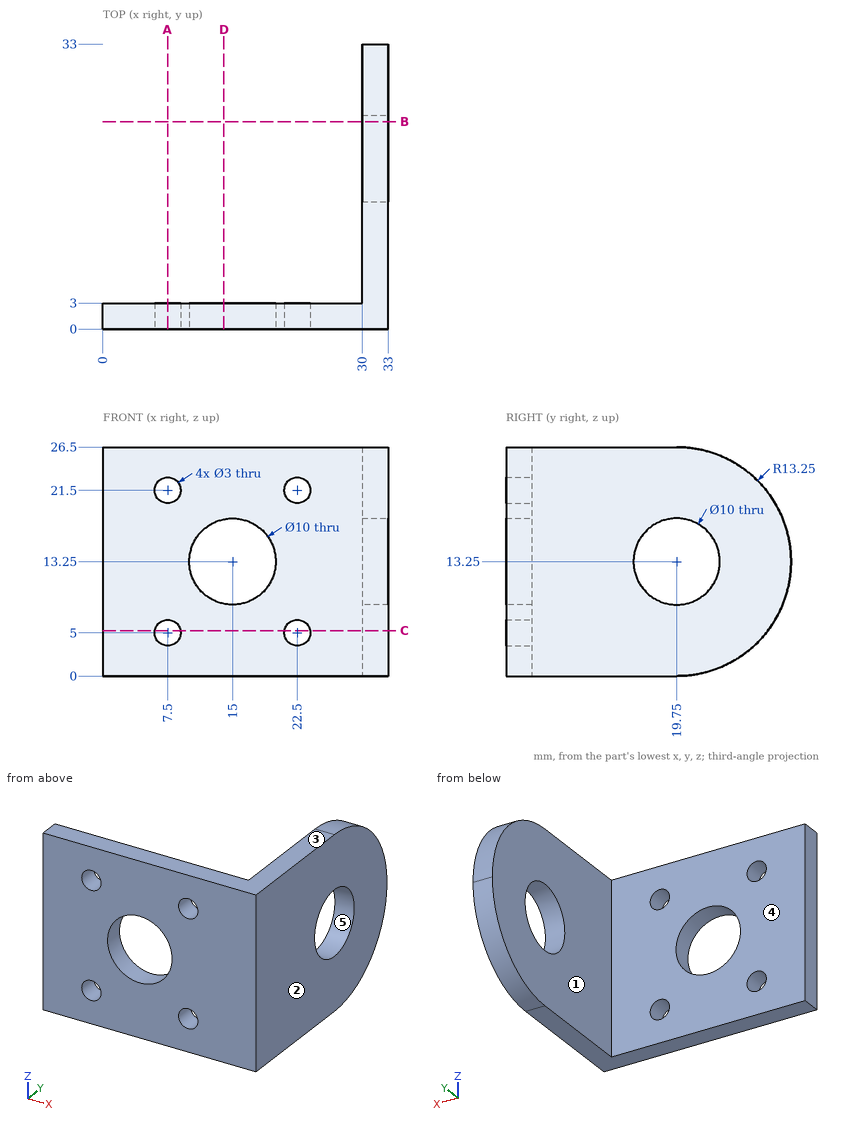
Part print with two shaded views. Sizes in mm from the minimum x, y, z corner. A direction names the side the tool comes from. Coordinates: 2 decimals unless noted, no trailing zeros. Write each loop counter-clockwise with the first axis right and the second up, starting at its lowest first coordinate (ties: lowest second). Pieces come first, ordered by that corner, then holes. Notation, with made-up numbers: (55.25, 68.25) - (70.25, 68.25) arc R16 cw to (70.25, 73.25) - close; hole circle Ø6 at (-20, 58). An arc over 180 degrees is marked (long way). Put each result on its own line as item: value.
1. Band-saw the part on D-D (x = 14). Write the cut outline in (y, z), then the cut area to 3 significant figures.
Final values:
outline: (0, 0) - (3, 0) - (3, 8.35) - (0, 8.35) - close; (0, 18.15) - (3, 18.15) - (3, 26.5) - (0, 26.5) - close
area: 50.1 mm²
2. Flat gauge pins, fed straight in: pin 1 Ø10 at (y, z) = (17, 11.5) entering from -X; pin 2 Ø8 at (y, z) = (19.75, 13.25) entering from -X; pin 3 Ø3 at (x, z) = (12, 8.5) entering from -Y; pin 4 Ø8 at (x, z) = (19.5, 10) entering from +Y. Where does each tip first touch, or does it go through?
Final values:
pin 1: stops at x = 30
pin 2: passes through
pin 3: stops at y = 0
pin 4: stops at y = 3
3. 3-axis set-ups, long thin cutter, end or side, ignore diameter. For the marked faces 1 and 2: which of +Z, -Z, +X, -X, +Y, -Y reach the whole face in a straight line?
Final values:
face 1: +Z, -Z, -X, +Y
face 2: +Z, -Z, +X, +Y, -Y
4. Two-plate mould, pull along Z, no slides. Class the marked faces 3, 4 and 5: +Z half, -Z half, draft (parallel to the pull), parting line (faces both ways), or undercut.
Final values:
face 3: +Z half
face 4: draft
face 5: undercut
5. Band-saw the part on C-C (z = 5.25). Write the cut outline in (x, y), then the cut area to 3 significant figures.
Final values:
outline: (0, 0) - (6.02, 0) - (6.02, 3) - (0, 3) - close; (8.98, 0) - (21.02, 0) - (21.02, 3) - (8.98, 3) - close; (23.98, 0) - (33, 0) - (33, 30.31) - (30, 30.31) - (30, 3) - (23.98, 3) - close
area: 163 mm²
6. Probe line 1 along X through (y, z) = (1.25, 13.25); line 2 along X through (y, z) = (1.35, 21.5); line 3 along Y through (x, z) = (7.5, 12). List the from-to ranges inside material, lowest first. Write a range as [from, to].
Final values:
line 1: x = [0, 10], [20, 33]
line 2: x = [0, 6], [9, 21], [24, 33]
line 3: y = [0, 3]
7. Band-saw the part on B-B (y = 24). Write the cut outline in (x, z), then the cut area to 3 significant figures.
Final values:
outline: (30, 0.7) - (33, 0.7) - (33, 10.62) - (30, 10.62) - close; (30, 15.88) - (33, 15.88) - (33, 25.8) - (30, 25.8) - close
area: 59.5 mm²
8. Band-saw the part on A-A (x = 7.5). Write the cut outline in (y, z), then the cut area to 3 significant figures.
Final values:
outline: (0, 0) - (3, 0) - (3, 3.5) - (0, 3.5) - close; (0, 6.5) - (3, 6.5) - (3, 20) - (0, 20) - close; (0, 23) - (3, 23) - (3, 26.5) - (0, 26.5) - close
area: 61.5 mm²
